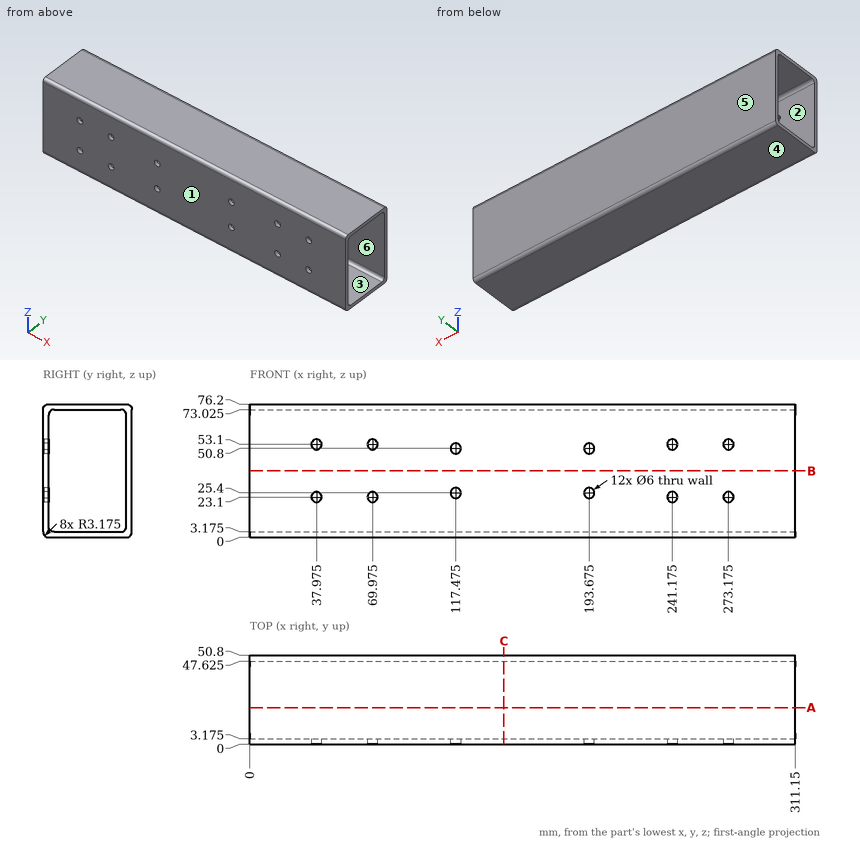
Verification items for this drawing (mm, ordinates from the low corner). A direction names the side the tool comes from. Coordinates: 2 decimals unless noted, no trailing zeros. Order: outer loops, then holes, each group sorted by start corner. A loop starts at its lowest first (then second) coordinate and runs counter-clockwise, first axis right, second up. Notation, with made-up numbers: (8, 78.25) -> (33, 78.25) arc R19 ccw to (33, 105.25) -> close; hole circle Ø4 at (79, -35.75). An arc over 180 degrees is marked (long way). Put each result on its own line as item: value. Start each with the question number.
1. Mould release check, pull along Z, two halves, no side actions. Record for the marked faces 3, 4, 5 and 6: released by +Z, released by -Z, zero draft, split by the parting line, or undercut.
2. Access from +Z, -Z, +X, -X, +Y, -Y to the whole of each face (thin tool, end or side, straight path). Record for the marked faces 1 and 2.
3. Go/stop test with a flat-tipped pin: pin 1 Ø5 at (x, z) = (241.175, 23.1) entering from -Y (3 decimals). Record where the tip stops, or that it passes through.
4. Cross-section at A-A, the plane y = 21. Record the boundary of the cut face in (x, z) (3 decimals), then the cut area to 3 significant figures.
5. Cross-section at B-B, the plane z = 38. Record the boundary of the cut face in (x, y) (3 decimals).
6. Cross-section at C-C, the plane x = 145. Record the boundary of the cut face in (y, z) (3 decimals), then the cut area to 3 significant figures.
7. Material ranges on L1, parallel to Z at x = 280, y = 40 (3 decimals); L2, parallel to Y at x = 24, z = 38 (3 decimals); L3, parallel to Y at x = 118.5, z = 28 (3 decimals), recorded low to high. Write a range as [from, to].
Computed:
1. face 3: undercut
1. face 4: released by -Z
1. face 5: zero draft
1. face 6: undercut
2. face 1: +Z, -Z, +X, -X, -Y
2. face 2: +X, -X
3. pin 1: y = 47.625
4. outline: (0, 0) -> (311.15, 0) -> (311.15, 3.175) -> (0, 3.175) -> close; (0, 73.025) -> (311.15, 73.025) -> (311.15, 76.2) -> (0, 76.2) -> close
4. area: 1,980 mm2
5. outline: (0, 0) -> (311.15, 0) -> (311.15, 3.175) -> (0, 3.175) -> close; (0, 47.625) -> (311.15, 47.625) -> (311.15, 50.8) -> (0, 50.8) -> close
6. outline: (0, 3.175) arc R3.175 ccw to (3.175, 0) -> (47.625, 0) arc R3.175 ccw to (50.8, 3.175) -> (50.8, 73.025) arc R3.175 ccw to (47.625, 76.2) -> (3.175, 76.2) arc R3.175 ccw to (0, 73.025) -> close; hole (3.175, 6.35) arc R3.175 ccw to (6.35, 3.175) -> (44.45, 3.175) arc R3.175 ccw to (47.625, 6.35) -> (47.625, 69.85) arc R3.175 ccw to (44.45, 73.025) -> (6.35, 73.025) arc R3.175 ccw to (3.175, 69.85) -> close
6. area: 766 mm2
7. L1: [0, 3.175], [73.025, 76.2]
7. L2: [0, 3.175], [47.625, 50.8]
7. L3: [47.625, 50.8]
